Geometry check sheet. Reference: the model listing, model coordinates, mm. A direction names the side the tool comes from. Give positions to 0.01 mm unless a question says otherwise; leave off trailing zeros. Loops run counter-clockwise (first coordinate to the right, second up) from the corner with the lowest first, then second, coordinate; pieces in that order, holes last. Notation, with made-up numbers: (10, 2) -> (15, 2) arc R15 ccw to (15, 24) -> close; hole circle Ø6 at (-34, 52.5). An arc over 180 degrees is marked (long way). One line per question, with ' | ' between items.
from build123d import *

# Parameters (mm, degrees)
BOSS_EXTRUDE1_DEPTH             = 20
CUT_EXTRUDE1_DEPTH              = 4
BOSS_EXTRUDE2_REACH             = 10.66
SKETCH4_R                       = 1
BOSS_EXTRUDE2_DIRECTION_2_REACH = 10.66


with BuildPart() as part:
    # Sketch1 → Boss-Extrude1 (new body)
    with BuildSketch(Plane(origin=(0, 0, 0), x_dir=(1, 0, 0), z_dir=(0, 1, 0))):
        Polygon((10, 0), (5, 8.660254038), (-5, 8.660254038), (-10, 0), (-5, -8.660254038), (5, -8.660254038), align=None)
    extrude(amount=BOSS_EXTRUDE1_DEPTH)

    # Sketch3 → Cut-Extrude1 (cut)
    with BuildSketch(Plane(origin=(0, 20, 0), x_dir=(1, 0, 0), z_dir=(0, 1, 0))):
        Polygon((4.422649731, -7.660254038), (8.845299462, 0), (4.422649731, 7.660254038), (-4.422649731, 7.660254038), (-8.845299462, 0), (-4.422649731, -7.660254038), align=None)
    extrude(amount=-CUT_EXTRUDE1_DEPTH, mode=Mode.SUBTRACT)

    # Sketch4 → Boss-Extrude2 (add, up to next)
    with BuildSketch(Plane.XY, mode=Mode.PRIVATE) as boss_extrude2_sk1:
        with Locations((0, 18)):
            Circle(SKETCH4_R)
    boss_extrude2_tool1 = extrude(boss_extrude2_sk1.sketch, amount=BOSS_EXTRUDE2_REACH, mode=Mode.PRIVATE) - part.part
    add(boss_extrude2_tool1.solids().sort_by_distance((0, 18, 0))[0])

    # Sketch4 → Boss-Extrude2 direction 2 (add, up to next)
    with BuildSketch(Plane.XY, mode=Mode.PRIVATE) as boss_extrude2_direction_2_sk1:
        with Locations((0, 18)):
            Circle(SKETCH4_R)
    boss_extrude2_direction_2_tool1 = extrude(boss_extrude2_direction_2_sk1.sketch, amount=-BOSS_EXTRUDE2_DIRECTION_2_REACH, mode=Mode.PRIVATE) - part.part
    add(boss_extrude2_direction_2_tool1.solids().sort_by_distance((0, 18, 0))[0])


solid = part.part
Item 1: Release check for a two-part mould opening along Z. For faces 3 (the face through (-7.465, 9.86, -4.391)), 4 (the face through (1, 20, -8)), 5 (the face through (1, 17, -7.66)), 6 (the face through (0, 16, 0)) record: pulls with the +Z half, pulls with the -Z half, needs draft (parallel to the pull), parting line crosses it, or undercut.
Result:
face 3: pulls with the -Z half | face 4: needs draft | face 5: undercut | face 6: undercut
Item 2: Sectioned sample at A-A (x = 0). Record the cut outline in (y, z), plus the area to 3 significant figures.
Result:
outline: (0, -8.66) -> (20, -8.66) -> (20, -7.66) -> (19, -7.66) -> (19, 7.66) -> (20, 7.66) -> (20, 8.66) -> (0, 8.66) -> close; hole (16, -7.66) -> (17, -7.66) -> (17, 7.66) -> (16, 7.66) -> close | area: 316 mm2
Item 3: Sectioned sample at B-B (y = 18). Record the cut outline in (x, z), plus the area to 3 significant figures.
Result:
outline: (-10, 0) -> (-5, -8.66) -> (5, -8.66) -> (10, 0) -> (5, 8.66) -> (-5, 8.66) -> close; hole (-8.85, 0) -> (-4.42, -7.66) -> (-1, -7.66) -> (-1, 7.66) -> (-4.42, 7.66) -> close; hole (1, -7.66) -> (4.42, -7.66) -> (8.85, 0) -> (4.42, 7.66) -> (1, 7.66) -> close | area: 87.2 mm2
Item 4: Scan lines: probe 1 along X at (y, z) = (17.25, 1.25); probe 2 along Y at (x, z) = (5.5, -4); probe 3 along Y at (x, z) = (-0.25, 0.75). Record each from-to range of solid material in increasing order.
Result:
probe 1: -9.28 to -8.12, -0.66 to 0.66, 8.12 to 9.28 | probe 2: 0 to 16 | probe 3: 0 to 16, 17.03 to 18.97
Item 5: Set-up check for faces 1 (the face through (-6.603, 18.028, -3.884)), 2 (the face through (0, 10, 8.66)): record each of +Z, -Z, +X, -X, +Y, -Y from which the full face is reachable in a straight line by a thin tool's end or side.
Result:
face 1: +Y | face 2: +Z, +X, -X, +Y, -Y
Item 6: Sectioned sample at D-D (x = 3.5). Record the cut outline in (y, z), plus the area to 3 significant figures.
Result:
outline: (0, -8.66) -> (20, -8.66) -> (20, -7.66) -> (16, -7.66) -> (16, 7.66) -> (20, 7.66) -> (20, 8.66) -> (0, 8.66) -> close | area: 285 mm2
Item 7: Sectioned sample at C-C (z = 7). Record the cut outline in (x, y), plus the area to 3 significant figures.
Result:
outline: (-5.96, 0) -> (5.96, 0) -> (5.96, 20) -> (4.8, 20) -> (4.8, 16) -> (-4.8, 16) -> (-4.8, 20) -> (-5.96, 20) -> close; circle Ø2 at (0, 18) | area: 203 mm2
Item 8: Depth check by flat-ended pin: pin 1 Ø2 at (y, z) = (2, -5) entering from +X; pin 2 Ø12 at (x, y) = (8, 6.5) entering from -Z; pin 3 Ø1.5 at (y, z) = (9, -3.5) entering from -X; pin 4 Ø5 at (y, z) = (17.5, -4) entering from +X. Enter the tip coordinate at first touch or a pass-through.
Result:
pin 1: x = 7.69 | pin 2: z = -8.66 | pin 3: x = -8.41 | pin 4: x = 9.13
